For this review, take the finished solid that the model builds, in its own axes (mm). A direction names the side the tool comes from. Round coordinates to 2 decimals unless told otherwise and drop trailing zeros. Write each loop counter-clockwise with the first axis right and the second up, starting at its lowest first coordinate (ties: lowest second). Pieces come first, ordered by that corner, then holes. Notation, with made-up numbers: M 51.25,89.5 L 96.25,89.5 A23 cw 96.25,126.5 Z; hole C -2.75,73.25 d1. An arc over 180 degrees is marked long. Use one line per item in the form item = value. Start each with the question number.
Item 1: Add section B-B (z = 13). State the section outline as (x, y) points.
Item 2: Draft analysis for pull direction Y (two halves, no side actions). For faces 1 (the flat face through (10, 0, 16)), 2 (the flat face through (12.5, 0, 14)), 3 (the flat face through (-9, -17.5, 25)), state which applies: released by +Y, released by -Y, zero draft, split by the parting line, or undercut.
Item 3: For faces 4 (the flat face through (10, 0, 44)), 5 (the flat face through (-12.5, 0, 14)), 6 (the flat face through (7.5, 0, 13)), 7 (the flat face through (7, 0, 2)), list the 3-axis set-ups (+Z, -Z, +X, -X, +Y, -Y) from which the entire face can be reached by the end or side of a thin tool; tool diameter is ignored.
Item 4: Add section D-D (y = -13.9). State the section outline as (x, z) points, and give its area (3 significant figures).
Item 5: Add section C-C (x = -6). State the section outline as (y, z) points.
Item 6: Add section A-A (y = 9). State the section outline as (x, z) points, and give its area (3 significant figures).
Item 7: For P1, Ø8, axis at x = 2, y = 12, coming from the +Z side; P2, Ø6, axis at x = 1.5, y = 0.5, coming from the -Z side, all flat-tipped, find the tip position at first contact; note any pin that passes through.
Item 8: For line 1 (Y direction, x = 11, z = 37); line 2 (X direction, y = 11, z = 13); line 3 (Z direction, x = 11.25, y = 6), list the stretches that pass through material, from the lowest coordinate up. Write a range as [from, to].
from build123d import *

# Parameters (mm, degrees)
SKETCH1_W           = 20
SKETCH1_H           = 35
SKETCH1_R           = 1
SKETCH1_W_2         = 14
SKETCH1_H_2         = 24
BOSS_EXTRUDE1_DEPTH = 5
SKETCH2_W           = 50
SKETCH2_H           = 35
BOSS_EXTRUDE2_DEPTH = 2.5
SKETCH3_R           = 1
SKETCH3_W           = 28
SKETCH3_H           = 24
CUT_EXTRUDE1_DEPTH  = 5


with BuildPart() as part:
    # Sketch1 → Boss-Extrude1 (new body)
    with BuildSketch(Plane.XY):
        Rectangle(SKETCH1_W, SKETCH1_H)
        with Locations((0, 13.9)):
            Circle(SKETCH1_R, mode=Mode.SUBTRACT)
        with Locations(Location((0, -13.9, 0), (0, 0, 180))):
            Circle(SKETCH1_R, mode=Mode.SUBTRACT)
        Rectangle(SKETCH1_W_2, SKETCH1_H_2, mode=Mode.SUBTRACT)
    extrude(amount=BOSS_EXTRUDE1_DEPTH)

    # Sketch2 → Boss-Extrude2 (add, symmetric)
    with BuildSketch(Plane(origin=(10, 0, 0), x_dir=(0, 0, -1), z_dir=(1, 0, 0))):
        with Locations((-25, 0)):
            Rectangle(SKETCH2_W, SKETCH2_H)
    boss_extrude2 = extrude(amount=BOSS_EXTRUDE2_DEPTH, both=True)

    # Sketch3 → Cut-Extrude1 (cut)
    with BuildSketch(Plane.ZY.offset(-7.5)):
        with Locations((23, 13.9)):
            Circle(SKETCH3_R)
        with Locations(Location((37, 13.9, 0), (0, 0, 180))):
            Circle(SKETCH3_R)
        with Locations((37, -13.9)):
            Circle(SKETCH3_R)
        with Locations(Location((23, -13.9, 0), (0, 0, 180))):
            Circle(SKETCH3_R)
        with Locations((30, 0)):
            Rectangle(SKETCH3_W, SKETCH3_H)
    cut_extrude1 = extrude(amount=-CUT_EXTRUDE1_DEPTH, mode=Mode.SUBTRACT)

    # Mirror2: Boss-Extrude2, Cut-Extrude1 across plane
    add(boss_extrude2.mirror(Plane.ZY))
    add(cut_extrude1.mirror(Plane.ZY), mode=Mode.SUBTRACT)


solid = part.part
Calculated:
q1.outline = M -12.5,-17.5 L -7.5,-17.5 L -7.5,17.5 L -12.5,17.5 Z; M 7.5,-17.5 L 12.5,-17.5 L 12.5,17.5 L 7.5,17.5 Z
q2.face_1 = undercut
q2.face_2 = zero draft
q2.face_3 = released by -Y
q3.face_4 = +X, -X
q3.face_5 = +Z, -Z, -X, +Y, -Y
q3.face_6 = +Z, +Y, -Y
q3.face_7 = +Z, -Z
q4.outline = M -12.5,0 L -1,0 L -1,5 L -7.5,5 L -7.5,22 L -12.5,22 Z; M -12.5,24 L -7.5,24 L -7.5,36 L -12.5,36 Z; M -12.5,38 L -7.5,38 L -7.5,50 L -12.5,50 Z; M 1,0 L 12.5,0 L 12.5,22 L 7.5,22 L 7.5,5 L 1,5 Z; M 7.5,24 L 12.5,24 L 12.5,36 L 7.5,36 Z; M 7.5,38 L 12.5,38 L 12.5,50 L 7.5,50 Z
q4.area = 525 mm^2
q5.outline = M -17.5,0 L -12,0 L -12,5 L -17.5,5 Z; M 12,0 L 17.5,0 L 17.5,5 L 12,5 Z
q6.outline = M -12.5,0 L -7,0 L -7,5 L -7.5,5 L -7.5,16 L -12.5,16 Z; M -12.5,44 L -7.5,44 L -7.5,50 L -12.5,50 Z; M 7,0 L 12.5,0 L 12.5,16 L 7.5,16 L 7.5,5 L 7,5 Z; M 7.5,44 L 12.5,44 L 12.5,50 L 7.5,50 Z
q6.area = 225 mm^2
q7.P1 = 5
q7.P2 = through
q8.line_1 = [-17.5, -14.9], [-12.9, -12], [12, 12.9], [14.9, 17.5]
q8.line_2 = [-12.5, -7.5], [7.5, 12.5]
q8.line_3 = [0, 16], [44, 50]
